```python
from build123d import *

# Parameters (mm, degrees)
F1_DEPTH = 5.6642


with BuildPart() as f1:
    # F0 (on Front) → F1 (new body)
    with BuildSketch(Plane.XZ):
        with BuildLine():
            Line((-39.6875, 0), (0, 0))
            Line((0, 0), (0, 4.145858))
            Line((0, 4.145858), (-42.1894, 4.145858))
            Line((-42.1894, 4.145858), (-44.198703, 4.145858))
            ThreePointArc((-44.198703, 4.145858), (-46.546897, 2.637402), (-47.4599, 0))
            Line((-47.4599, 0), (-44.6913, 0))
            ThreePointArc((-44.6913, 0), (-42.1894, 2.5019), (-39.6875, 0))
        make_face()
        with BuildLine():
            Line((0, -4.145858), (0, 0))
            Line((0, 0), (-39.6875, 0))
            ThreePointArc((-39.6875, 0), (-42.1894, -2.5019), (-44.6913, 0))
            Line((-44.6913, 0), (-47.4599, 0))
            ThreePointArc((-47.4599, 0), (-46.546897, -2.637402), (-44.198703, -4.145858))
            Line((-44.198703, -4.145858), (-42.1894, -4.145858))
            Line((-42.1894, -4.145858), (0, -4.145858))
        make_face()
        with BuildLine():
            ThreePointArc((39.6875, 0), (42.1894, 2.5019), (44.6913, 0))
            Line((44.6913, 0), (47.4599, 0))
            ThreePointArc((47.4599, 0), (46.546897, 2.637402), (44.198703, 4.145858))
            Line((44.198703, 4.145858), (42.1894, 4.145858))
            Line((42.1894, 4.145858), (0, 4.145858))
            Line((0, 4.145858), (0, 0))
            Line((0, 0), (39.6875, 0))
        make_face()
        with BuildLine():
            Line((47.4599, 0), (44.6913, 0))
            ThreePointArc((44.6913, 0), (42.1894, -2.5019), (39.6875, 0))
            Line((39.6875, 0), (0, 0))
            Line((0, 0), (0, -4.145858))
            Line((0, -4.145858), (42.1894, -4.145858))
            Line((42.1894, -4.145858), (44.198703, -4.145858))
            ThreePointArc((44.198703, -4.145858), (46.546897, -2.637402), (47.4599, 0))
        make_face()
    extrude(amount=F1_DEPTH)


solid = f1.part
```
Could you check a few things on this model? Use its own coordinates, in mm. Round coordinates to 2 decimals unless told otherwise and drop trailing zeros. Write each loop counter-clockwise with the first axis right and the second up, starting at its lowest first coordinate (ties: lowest second). Pieces come first, ordered by that corner, then holes. Notation, with made-up numbers: M 19.5,61.5 L 60.5,61.5 A15 ccw 60.5,68.5 Z; hole C 4.25,26 d3. An arc over 180 degrees is marked long. Write each question's results on one line, items separated by ' | '. Start each with the question number.
1. Imagine slicing it at A-A on y = -0.85. List the corners of the cut face in (x, z) for me.
2. Thinking about a two-plate mould opening in Z: for faces 1 (the face through (1, -3, 4.146)), 2 (the face through (-1, -3, -4.146)), 3 (the face through (-39.803, -2.792, -0.752)), 4 (the face through (44.576, -2.792, -0.752)), which applies, +Z half, -Z half, draft (parallel to the pull), parting line (faces both ways), or undercut?
3. I'm going to push flat-ended pins straight in: pin 1 Ø1 at (y, z) = (-2, 3) entering from +X; pin 2 Ø4 at (x, z) = (-42.19, 0) entering from +Y. Where does each tip first touch, or does it pass through?
4. I need wall thicknesses on L1, parallel to X at y = -0.55, z = -1; L2, parallel to Z at x = -42.5, y = -5.1; L3, parallel to X at y = -5.3, z = -0.75. Which ranges of each line are inside material? Lowest first, please. Write a range as from..to.
Result sheet:
1) outline: M -44.2,-4.15 L 44.2,-4.15 A4.27 ccw 44.2,4.15 L -44.2,4.15 A4.27 ccw Z; hole C -42.19,0 d5; hole C 42.19,0 d5
2) face 1: +Z half | face 2: -Z half | face 3: undercut | face 4: undercut
3) pin 1: stops at x = 46.65 | pin 2: passes through
4) L1: x = -47.34..-44.48, -39.9..39.9, 44.48..47.34 | L2: z = -4.15..-2.48, 2.48..4.15 | L3: x = -47.39..-44.58, -39.8..39.8, 44.58..47.39
